Can you work these out from the model? Positions are in its coordinate system, mm. A direction names the side the tool comes from. Give positions to 0.01 mm unless a question says otherwise; leave off trailing zeros. Order: outer loops, then holes, each group sorted by start corner. A loop starts at its lowest first (then second) coordinate and runs counter-clockwise, first axis right, second up. Notation, with made-up numbers: (79, 58) - (136, 58) arc R20 ccw to (136, 68) - close; hole circle Ø8 at (15, 37.5). An arc over 180 degrees is marked (long way). Answer as a JSON object with one key per item and string values.
Autodesk Inventor part; units mm, degrees
ref_plane "YZ Plane" through (0, 0, 0) normal (1, 0, 0) x (0, 1, 0)
ref_plane "XZ Plane" through (0, 0, 0) normal (0, 1, 0) x (-1, 0, 0)
ref_plane "XY Plane" through (0, 0, 0) normal (0, 0, 1) x (1, 0, 0)
sketch "Esquisse1" plane through (0, 0, 0) normal (0, 1, 0) x (-1, 0, 0)
  line L0 (0, -308) -> (0, 308) construction
  line L1 (-119, 0) -> (119, 0) construction
  line L2 (-85, -220) -> (85, -220)
  line L3 (85, -220) -> (85, 220)
  line L4 (85, 220) -> (-85, 220)
  line L5 (-85, 220) -> (-85, -220)
  line L6 (-85, -220) -> (85, 220) construction
  line L7 (85, -220) -> (-85, 220) construction
  point P0 (0, 0)
  dimension "d0" = 170
  dimension "d1" = 440
extrude "Extrusion1" add sketch "Esquisse1" along normal mid plane 70
fillet "Congé1" radius 5 4 edges at (85, -35, 0) (85, 35, 0) (-85, -35, 0) (-85, 35, 0)
sketch "Sketch2" plane through (80, 35, -220) normal (0, 0, -1) x (-1, 0, 0)
  arc A0 (165, -5) -> (160, 0) centre (160, -5) ccw construction
  line L0 (0, 0) -> (160, 0) construction
  arc A1 (0, 0) -> (-5, -5) centre (0, -5) ccw construction
  line L1 (-5, -5) -> (-5, -65) construction
  arc A2 (-5, -65) -> (0, -70) centre (0, -65) ccw construction
  line L2 (160, -70) -> (0, -70) construction
  arc A3 (160, -70) -> (165, -65) centre (160, -65) ccw construction
  line L3 (165, -65) -> (165, -5) construction
  arc A4 (-3, -65) -> (0, -68) centre (0, -65) ccw
  line L4 (-3, -65) -> (-3, -5)
  arc A5 (0, -2) -> (-3, -5) centre (0, -5) ccw
  line L5 (0, -2) -> (160, -2)
  arc A6 (163, -5) -> (160, -2) centre (160, -5) ccw
  line L6 (163, -5) -> (163, -65)
  arc A7 (160, -68) -> (163, -65) centre (160, -65) ccw
  line L7 (160, -68) -> (0, -68)
  point P0 (80, -35)
  dimension "d5" = 2
extrude "Extrusion2" cut sketch "Sketch2" against normal through all
properties part number "Casing_Generator"
Q1. I need wall thicknesses on L1, parallel to Y at x = 17, z = -22; L2, parallel to X at y = -0.5, z = -26. Which ranges of each line are inside material? Lowest first, please.
Recorded:
{"L1": "y = -35 to -33, 33 to 35", "L2": "x = -85 to -83, 83 to 85"}
Q2. Which directions (+Z, -Z, +X, -X, +Y, -Y) give clear straight access to the entire face, cutting with the end or side of a thin tool? Please do faces 4 (the face through (0, -34, -220)), 5 (the face through (-1, -33, -3)).
Recorded:
{"face 4": "-Z, +X, -X, +Y, -Y", "face 5": "+Z, -Z"}
Q3. If we section it at A-A, the plane y = 4: Please give me the cut outline in (x, z), then the cut area to 3 significant figures.
Recorded:
{"outline": "(-85, -220) - (-83, -220) - (-83, 220) - (-85, 220) - close; (83, -220) - (85, -220) - (85, 220) - (83, 220) - close", "area": "1,760 mm^2"}
Q4. If we section it at B-B, the plane x = 70: Please give me the cut outline in (y, z).
Recorded:
{"outline": "(-35, -220) - (-33, -220) - (-33, 220) - (-35, 220) - close; (33, -220) - (35, -220) - (35, 220) - (33, 220) - close"}
Q5. We'd pull the mould along X, two halves only. Please class faces 1 (the face through (85, 0, 3)), 2 (the face through (1, -35, 3)), 3 (the face through (1, 33, -3)): released by +X, released by -X, zero draft, split by the parting line, or undercut.
Recorded:
{"face 1": "released by +X", "face 2": "zero draft", "face 3": "undercut"}
Q6. If we section it at C-C, the plane z = 87: Please give me the cut outline in (x, y).
Recorded:
{"outline": "(-85, -30) arc R5 ccw to (-80, -35) - (80, -35) arc R5 ccw to (85, -30) - (85, 30) arc R5 ccw to (80, 35) - (-80, 35) arc R5 ccw to (-85, 30) - close; hole (-83, -30) arc R3 ccw to (-80, -33) - (80, -33) arc R3 ccw to (83, -30) - (83, 30) arc R3 ccw to (80, 33) - (-80, 33) arc R3 ccw to (-83, 30) - close"}
